```python
from build123d import *

# Parameters (mm, degrees)
F0_R     = 3
F0_R_2   = 2.75
F0_R_3   = 1.5
F1_DEPTH = 1


# Not quite as in the source:
# - ends of sketch curves that miss each other by under 0.0002 mm in the source are joined


with BuildPart() as f1:
    # F0 (on Front) → F1 (new body)
    with BuildSketch(Plane.XZ):
        with BuildLine():
            ThreePointArc((10.2610980266, 73.2851271902), (13.0931802752, 72.8324696154), (15.9055950445, 72.2704092024))
            Line((15.9055950445, 72.2704092024), (16.286797, 73.722386))
            Line((16.286797, 73.722386), (22.888167, 98.86666))
            Line((22.888167, 98.86666), (22.234036, 104.134663))
            ThreePointArc((22.234036, 104.134663), (-14.4021915305, 105.5033516635), (-49.3311389264, 94.3653488593))
            Line((-49.3311389264, 94.3653488593), (-48.548236, 89.117403))
            Line((-48.548236, 89.117403), (-35.435226, 66.667794))
            Line((-35.435226, 66.667794), (-34.67805, 65.371499))
            ThreePointArc((-34.67805, 65.371499), (-22.8153047874, 70.3950414977), (-10.2610980266, 73.2851271902))
            ThreePointArc((-10.2610980266, 73.2851271902), (-8.0030918925, 71.581775015), (-9.706443985, 69.3237688925))
            ThreePointArc((-9.706443985, 69.3237688925), (-11.056110798, 69.1213600418), (-12.4015749915, 68.8926769529))
            ThreePointArc((-12.4015749915, 68.8926769529), (-13.6918696678, 68.5193918089), (-14.8778891297, 67.8888681928))
            ThreePointArc((-14.8778891297, 67.8888681928), (-17.7216913701, 63.1014792158), (-15.8160679868, 57.8693760134))
            ThreePointArc((-15.8160679868, 57.8693760134), (-13.6269577418, 58.088804993), (-11.5555822107, 57.3473496681))
            ThreePointArc((-11.5555822107, 57.3473496681), (-7.6357821132, 57.9995244077), (-3.6807509947, 58.3840909162))
            ThreePointArc((-3.6807509947, 58.3840909162), (0, 60), (3.6807510132, 58.3840910122))
            ThreePointArc((3.6807510132, 58.3840910122), (7.6357821132, 57.9995244077), (11.5555819538, 57.3473497706))
            ThreePointArc((11.5555819538, 57.3473497706), (13.6269577418, 58.088804993), (15.8160679296, 57.8693757888))
            ThreePointArc((15.8160679296, 57.8693757888), (17.7216913701, 63.1014792158), (14.8778891297, 67.8888681928))
            ThreePointArc((14.8778891297, 67.8888681928), (13.6918696678, 68.5193918089), (12.4015750198, 68.8926771098))
            ThreePointArc((12.4015750198, 68.8926771098), (11.056110798, 69.1213600418), (9.7064439965, 69.3237689753))
            ThreePointArc((9.7064439965, 69.3237689753), (8.0030918925, 71.581775015), (10.2610980266, 73.2851271902))
        make_face()
        with Locations((-11.25, 62.4955)):
            Circle(F0_R, mode=Mode.SUBTRACT)
        with Locations((-24.770679, 89.121622)):
            Circle(F0_R_2, mode=Mode.SUBTRACT)
        with Locations((0, 81.481831)):
            Circle(F0_R_3, mode=Mode.SUBTRACT)
        with Locations((0, 92.5)):
            Circle(F0_R_2, mode=Mode.SUBTRACT)
        with Locations((11.25, 62.4955)):
            Circle(F0_R, mode=Mode.SUBTRACT)
    extrude(amount=F1_DEPTH)


solid = f1.part
```
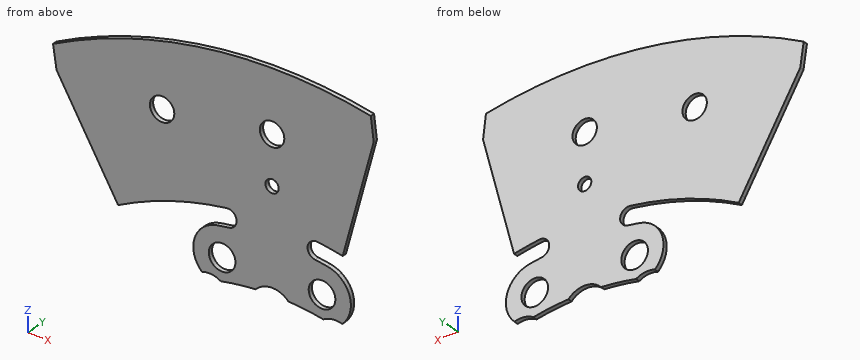
Geometry check sheet. Reference: the model listing, model coordinates, mm. Round coordinates to 2 decimals unless told otherwise and drop trailing zeros. Order: outer loops, then holes, each group sorted by start corner. A loop starts at its lowest first (then second) coordinate and runs counter-clockwise, first axis right, second up. Notation, with made-up numbers: (-33.75, -17) - (6.25, -17) arc R17 cw to (6.25, 0) - close; hole circle Ø4 at (0.25, 45). An arc over 180 degrees is marked (long way). Use a Markdown table: item, result. Add a question column.
1) Thickness scan on line 1 along Z through (x, y) = (0, -0.7); line 2 along Z through (x, y) = (-11.25, -0.6); line 3 along X through (y, z) = (-0.6, 90.5). Record the ranges inside material, lowest first.
2) Section check A-A (x = 0). Record the cut outline in (y, z), then the cut area to 3 significant figures.
3) Section check C-C (y = -0.8). Record the cut outline in (x, z).
4) Section check B-B (x = -17). Record the cut outline in (y, z).
5) Section check D-D (z = 102). Record the cut outline in (x, y).
Established:
| question | item | result |
|---|---|---|
| 1 | line 1 | 60 to 79.98, 82.98 to 89.75, 95.25 to 106.48 |
| 1 | line 2 | 57.41 to 59.5, 65.5 to 69.09, 73.14 to 105.89 |
| 1 | line 3 | -48.75 to -27.15, -22.39 to -1.89, 1.89 to 20.69 |
| 2 | outline | (-1, 60) - (0, 60) - (0, 79.98) - (-1, 79.98) - close; (-1, 82.98) - (0, 82.98) - (0, 89.75) - (-1, 89.75) - close; (-1, 95.25) - (0, 95.25) - (0, 106.48) - (-1, 106.48) - close |
| 2 | area | 38.0 mm2 |
| 3 | outline | (-49.33, 94.37) - (-48.55, 89.12) - (-35.44, 66.67) - (-34.68, 65.37) arc R74 cw to (-10.26, 73.29) arc R2 cw to (-9.71, 69.32) arc R70 ccw to (-12.4, 68.89) arc R6.5 ccw to (-14.88, 67.89) arc R6.5 ccw to (-15.82, 57.87) arc R5 cw to (-11.56, 57.35) arc R58.5 cw to (-3.68, 58.38) arc R5 cw to (3.68, 58.38) arc R58.5 cw to (11.56, 57.35) arc R5 cw to (15.82, 57.87) arc R6.5 ccw to (12.4, 68.89) arc R70 ccw to (9.71, 69.32) arc R2 cw to (10.26, 73.29) arc R74 cw to (15.91, 72.27) - (16.29, 73.72) - (22.89, 98.87) - (22.23, 104.13) arc R106.48 ccw to start; hole circle Ø5.5 at (-24.77, 89.12); hole circle Ø6 at (-11.25, 62.5); hole circle Ø5.5 at (0, 92.5); hole circle Ø3 at (0, 81.48); hole circle Ø6 at (11.25, 62.5) |
| 4 | outline | (-1, 59.46) - (0, 59.46) - (0, 65.53) - (-1, 65.53) - close; (-1, 72.02) - (0, 72.02) - (0, 105.12) - (-1, 105.12) - close |
| 5 | outline | (-30.57, -1) - (22.5, -1) - (22.5, 0) - (-30.57, 0) - close |
